Can you work these out from the drawing? Everything is in mm from the part's minimum corner. A direction names the side the tool comes from. Give positions to 0.01 mm unless a question says otherwise; leave off trailing zeros. Order: outer loops, then holes, each group sorted by start corner. A loop starts at its lowest first (then second) coordinate and runs counter-clockwise, first axis right, second up. Notation, with made-up numbers: M -34.75,-16 L -24.75,-16 A13 ccw -24.75,-1 Z; hole C -3.5,35.25 d8. An arc over 180 degrees is marked long. Answer as a JSON object with one key per item and string values.
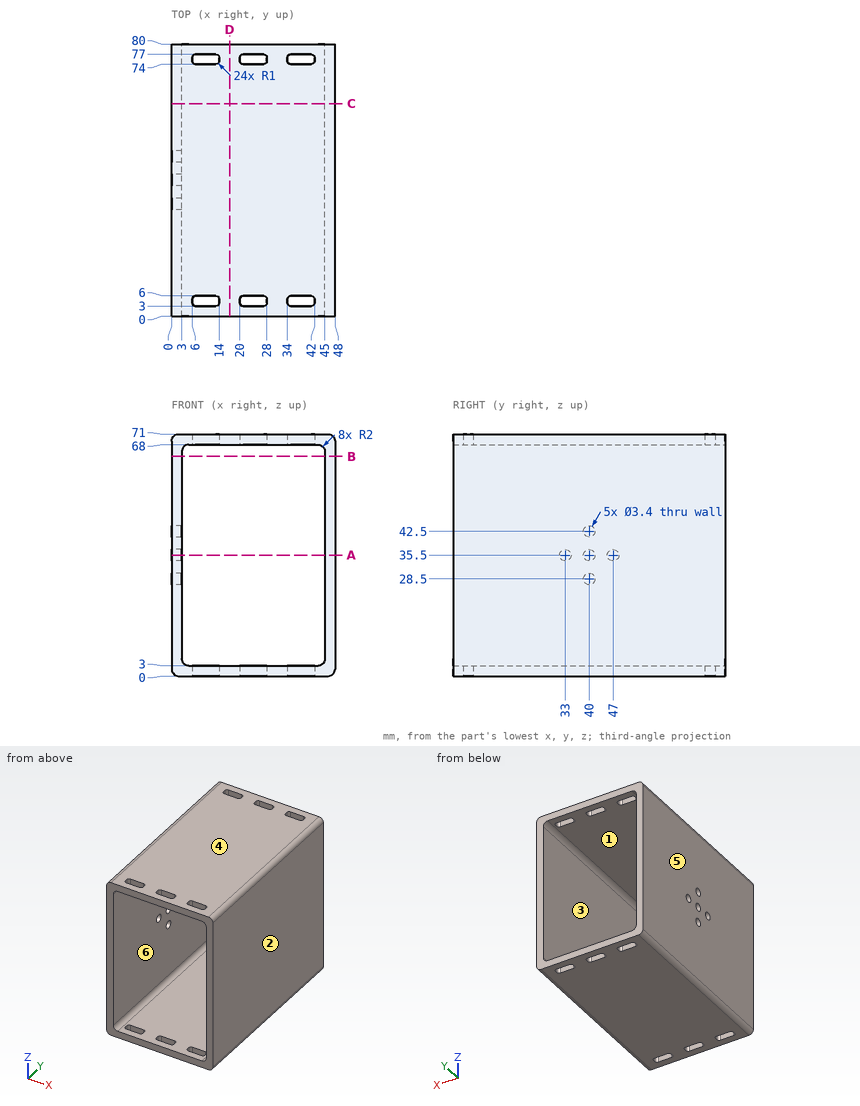
1) I'm going to push a flat-ended pin straight in: pin 1 Ø0.8 at (y, z) = (4.5, 1.5) entering from -X. Where does the tip first touch, or does it pass through?
Results found:
{"pin 1": "stops at x = 0"}
2) I want a section at D-D on x = 17. Write out the boundary of the cut face in (y, z).
Results found:
{"outline": "M 0,0 L 80,0 L 80,3 L 0,3 Z; M 0,68 L 80,68 L 80,71 L 0,71 Z"}
3) For the marked faces 1 and 2, which set-ups out of +Z, -Z, +X, -X, +Y, -Y let a thin tool reach every point of the face, with its end or its side?
Results found:
{"face 1": "+Y, -Y", "face 2": "+Z, -Z, +X, +Y, -Y"}
4) I want a section at A-A on z = 35.5. Write out the boundary of the cut face in (x, y).
Results found:
{"outline": "M 0,0 L 3,0 L 3,31.3 L 0,31.3 Z; M 0,34.7 L 3,34.7 L 3,38.3 L 0,38.3 Z; M 0,41.7 L 3,41.7 L 3,45.3 L 0,45.3 Z; M 0,48.7 L 3,48.7 L 3,80 L 0,80 Z; M 45,0 L 48,0 L 48,80 L 45,80 Z"}
5) Thinking about a two-plate mould opening in Z: for the marked faces 3, 4, 5 and 6, which applies, pulls with the +Z half, pulls with the -Z half, needs draft (parallel to the pull), parting line crosses it, or undercut?
Results found:
{"face 3": "undercut", "face 4": "pulls with the +Z half", "face 5": "needs draft", "face 6": "undercut"}
6) I need wall thicknesses on L1, parallel to Y at x = 1.8, z = 35.5; L2, parallel to Z at x = 39, y = 53.5; L3, parallel to X at y = 63, z = 65. Which ranges of each line are inside material? Lowest first, please.
Results found:
{"L1": "y = 0 to 31.3, 34.7 to 38.3, 41.7 to 45.3, 48.7 to 80", "L2": "z = 0 to 3, 68 to 71", "L3": "x = 0 to 3, 45 to 48"}
7) I want a section at C-C on y = 62.5. Write out the boundary of the cut face in (x, z), and give its area (3 significant figures).
Results found:
{"outline": "M 0,2 A2 ccw 2,0 L 46,0 A2 ccw 48,2 L 48,69 A2 ccw 46,71 L 2,71 A2 ccw 0,69 Z; hole M 3,5 A2 ccw 5,3 L 43,3 A2 ccw 45,5 L 45,66 A2 ccw 43,68 L 5,68 A2 ccw 3,66 Z", "area": "678 mm²"}
8) I want a section at B-B on z = 64.5. Write out the boundary of the cut face in (x, y), and give its area (3 significant figures).
Results found:
{"outline": "M 0,0 L 3,0 L 3,80 L 0,80 Z; M 45,0 L 48,0 L 48,80 L 45,80 Z", "area": "480 mm²"}
